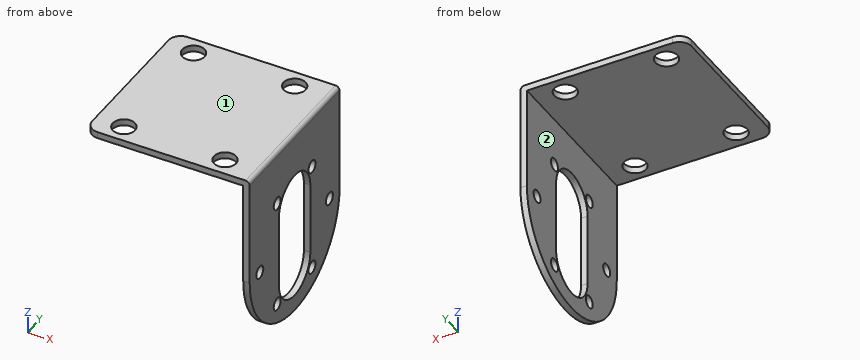
Autodesk Inventor part; units mm, degrees
ref_plane "작업 평면1" through (0, 0, 0) normal (0, 0, 1) x (1, 0, 0)
ref_plane "YZ Plane" through (0, 0, 0) normal (1, 0, 0) x (0, 1, 0)
ref_plane "XZ Plane" through (0, 0, 0) normal (0, 1, 0) x (-1, 0, 0)
ref_plane "작업 평면1" through (0, 0, 0) normal (0, 0, 1) x (1, 0, 0)
sketch "스케치1" plane through (0, 0, 0) normal (0, 0, 1) x (1, 0, 0)
  line L0 (130, -172.5) -> (91, -172.5)
  line L1 (91, -172.5) -> (91, -132.5)
  line L2 (91, -132.5) -> (130, -132.5)
  line L3 (130, -132.5) -> (130, -172.5)
  line L4 (91, -152.5) -> (130, -152.5) construction
  circle A0 centre (98, -168) radius 2.75
  line L5 (110.5, -172.5) -> (110.5, -132.5) construction
  circle A1 centre (98, -137) radius 2.75
  circle A2 centre (123, -168) radius 2.75
  circle A3 centre (123, -137) radius 2.75
  circle A4 centre (0, 170) radius 2
  circle A5 centre (-73.6122, 42.5) radius 2
  circle A6 centre (73.6122, 42.5) radius 2
  line L6 (-175, 220) -> (-175, 200)
  line L7 (-175, 200) -> (-130, 200)
  line L8 (-130, 200) -> (-130, 105)
  line L9 (-130, 105) -> (-175, 105)
  line L10 (-175, 105) -> (-175, -105)
  line L11 (-175, -105) -> (-130, -105)
  line L12 (-130, -105) -> (-130, -200)
  line L13 (-130, -200) -> (-175, -200)
  line L14 (-175, -200) -> (-175, -220)
  arc A7 (-175, -220) -> (-145, -250) centre (-145, -220) ccw
  line L15 (-145, -250) -> (145, -250)
  arc A8 (145, -250) -> (175, -220) centre (145, -220) ccw
  line L16 (175, -220) -> (175, -200)
  line L17 (175, -200) -> (130, -200)
  line L18 (130, -200) -> (130, -105)
  line L19 (130, -105) -> (175, -105)
  line L20 (175, -105) -> (175, 105)
  line L21 (175, 105) -> (130, 105)
  line L22 (130, 105) -> (130, 200)
  line L23 (130, 200) -> (175, 200)
  line L24 (175, 200) -> (175, 220)
  arc A9 (175, 220) -> (145, 250) centre (145, 220) ccw
  line L25 (145, 250) -> (-145, 250)
  arc A10 (-145, 250) -> (-175, 220) centre (-145, 220) ccw
  circle A11 centre (-123, 166.7672) radius 2
  circle A12 centre (122.9975, 135.7594) radius 2
  circle A13 centre (97.9975, -135.761) radius 2
  circle A14 centre (15.5, 71.3) radius 2
  circle A15 centre (165.0067, -210) radius 2.5
  circle A16 centre (119.0003, -180.2596) radius 1.25
  circle A17 centre (-119, -122.2672) radius 1.25
  circle A18 centre (-123, -135.7672) radius 2
  circle A19 centre (0.0196, 140) radius 2
  circle A20 centre (-123, -166.7672) radius 2
  circle A21 centre (-70, -122.2672) radius 1.25
  circle A22 centre (69.9966, -122.2627) radius 1.25
  circle A23 centre (-165, 0) radius 2.5
  circle A24 centre (-165.0067, 210) radius 2.5
  circle A25 centre (-15.5, 119.1) radius 2
  circle A26 centre (97.9995, -166.761) radius 2
  circle A27 centre (97.9995, 166.761) radius 2
  circle A28 centre (-98, 166.7672) radius 2
  circle A29 centre (-123, 135.7672) radius 2
  circle A30 centre (97.9975, 135.761) radius 2
  circle A31 centre (122.9975, -135.7594) radius 2
  circle A32 centre (-15.5, 71.3) radius 2
  circle A33 centre (-164.9933, -210) radius 2.5
  circle A34 centre (70.0003, -180.2627) radius 1.25
  circle A35 centre (-119, -180.2672) radius 1.25
  circle A36 centre (-98, -135.7672) radius 2
  circle A37 centre (47.6216, 57.483) radius 2
  circle A38 centre (-47.6412, 57.517) radius 2
  circle A39 centre (-98, -166.7672) radius 2
  circle A40 centre (-70, -180.2672) radius 1.25
  circle A41 centre (118.9966, -122.2596) radius 1.25
  circle A42 centre (165, 0) radius 2.5
  circle A43 centre (164.9933, 210) radius 2.5
  circle A44 centre (15.5, 119.1) radius 2
  circle A45 centre (122.9995, -166.7594) radius 2
  circle A46 centre (122.9995, 166.7594) radius 2
  circle A47 centre (-98, 135.7672) radius 2
  line L26 (-110, 97.5) -> (-93, 97.5)
  line L27 (-93, 97.5) -> (-93, 89.5)
  line L28 (-93, 89.5) -> (-110, 89.5)
  line L29 (-110, 89.5) -> (-110, 97.5)
  circle A48 centre (148, -23.75) radius 2
  circle A49 centre (130.626, -27.584) radius 1.5
  circle A50 centre (118.5, 61.5) radius 1.5
  circle A51 centre (-118.5, 61.5) radius 1.5
  circle A52 centre (21, -158.9548) radius 2
  circle A53 centre (-22, -53) radius 2
  circle A54 centre (-49.5, -194.9548) radius 2
  circle A55 centre (-49.5, -158.9548) radius 2
  circle A56 centre (21, -194.9548) radius 2
  circle A57 centre (-155, 25) radius 1.5
  circle A58 centre (118.5, 25) radius 1.5
  circle A59 centre (123.133, -76) radius 1.5
  circle A60 centre (37, -84) radius 2
  line L30 (-93, -89.5) -> (-93, -97.5)
  line L31 (-93, -97.5) -> (-110, -97.5)
  line L32 (-110, -97.5) -> (-110, -89.5)
  line L33 (-110, -89.5) -> (-93, -89.5)
  circle A61 centre (-130, 5) radius 6
  line L34 (110, 89.5) -> (93, 89.5)
  line L35 (93, 89.5) -> (93, 97.5)
  line L36 (93, 97.5) -> (110, 97.5)
  line L37 (110, 97.5) -> (110, 89.5)
  circle A62 centre (148, -84) radius 2
  circle A63 centre (47.999, -27.584) radius 1.5
  circle A64 centre (155, 61.5) radius 1.5
  circle A65 centre (-155, 61.5) radius 1.5
  circle A66 centre (49.5, -158.9548) radius 2
  circle A67 centre (-86, -93.5) radius 2
  circle A68 centre (-21, -194.9548) radius 2
  circle A69 centre (-150, -53) radius 2
  circle A70 centre (-21, -158.9548) radius 2
  circle A71 centre (49.5, -194.9548) radius 2
  circle A72 centre (-118.5, 25) radius 1.5
  circle A73 centre (155, 25) radius 1.5
  circle A74 centre (48, -76) radius 1.5
  circle A75 centre (37, -23.75) radius 2
  line L38 (110, -89.5) -> (110, -97.5)
  line L39 (110, -97.5) -> (93, -97.5)
  line L40 (93, -97.5) -> (93, -89.5)
  line L41 (93, -89.5) -> (110, -89.5)
  circle A76 centre (-70, 5) radius 6
  circle A77 centre (0, -216.4634) radius 1.5
  circle A78 centre (28.4775, -136.4634) radius 1.5
  circle A79 centre (-28.4775, -136.4634) radius 1.5
  point P0 (0, 0)
  dimension "d0" = 40
  dimension "d1" = 39
  dimension "d5" = 5.5
  dimension "d6" = 7
  dimension "d7" = 4.5
  dimension "d22" = 97.5
extrude "돌출1" add sketch "스케치1" along normal blind 1.6 contours L0 L1 L2 L3 | A0 A26 | A1 A13 | A2 A45 | A3 A31 picked at (98.3703, -165.1311) picked at (98.3657, -134.1305) picked at (122.627, -165.1309) picked at (123.3661, -134.13)
sketch "스케치2" plane through (130, -172.5, 0) normal (1, 0, 0) x (0, 0, -1)
  line L0 (0, 40) -> (-1.6, 40)
  line L1 (-1.6, 0) -> (25.4, 0)
  line L2 (45.4, 20) -> (45.4, 20)
  line L3 (25.4, 40) -> (-1.6, 40)
  line L4 (-1.6, 40) -> (-1.6, 0)
  arc A0 (25.4, 0) -> (45.4, 20) centre (25.4, 20) ccw
  arc A1 (45.4, 20) -> (25.4, 40) centre (25.4, 20) ccw
  circle A2 centre (25.4, 35.5) radius 1.55
  circle A3 centre (11.9766, 27.75) radius 1.55
  circle A4 centre (11.9766, 12.25) radius 1.55
  circle A5 centre (25.4, 4.5) radius 1.55
  circle A6 centre (38.8234, 12.25) radius 1.55
  circle A7 centre (38.8234, 27.75) radius 1.55
  line L5 (34.4, 20) -> (16.4, 20) construction
  line L6 (34.4, 27) -> (16.4, 27)
  line L7 (16.4, 13) -> (34.4, 13)
  arc A8 (34.4, 13) -> (34.4, 27) centre (34.4, 20) ccw
  arc A9 (16.4, 27) -> (16.4, 13) centre (16.4, 20) ccw
  line L8 (0, 40) -> (-1.6, 40)
  point P0 (0, 172.5)
  point P1 (45.4, 40)
  point P2 (45.4, 20)
  point P3 (-1.6, 40)
  point P4 (0, 40)
  dimension "d3" = 1.6
  dimension "d8" = 47
  dimension "d9" = 20
  dimension "d10" = 3.1
  dimension "d11" = 15.5
  dimension "d14" = 360
  dimension "d16" = 9
  dimension "d17" = 14
extrude "돌출2" add sketch "스케치2" along normal blind 1.6
fillet "모깎기1" radius 3 2 edges at (91, -132.5, 0.8) (91, -172.5, 0.8)
fillet "모깎기2" radius 1 1 edges at (131.6, -152.5, 1.6)
properties part number "SAFRS-P-0038"
Geometry: final body of the model. Coordinates: model frame, mm. Face numbers are marked on the shaded views. A direction names the side the tool comes from. Give positions to 0.01 mm unless a question says otherwise; leave off trailing zeros. Order: outer loops, then holes, each group sorted by start corner. A loop starts at its lowest first (then second) coordinate and runs counter-clockwise, first axis right, second up. Notation, with made-up numbers: (47, 48.25) -> (56, 48.25) arc R21 cw to (56, 70.25) -> close; hole circle Ø9 at (-28, 20). An arc over 180 degrees is marked (long way). Write each question's results on one line, items separated by ' | '. Start each with the question number.
1) Section A-A (x = 123). Return loops of the section in (y, z), then the cut area to 3 significant figures.
2) Section D-D (y = -161). Return loops of the section in (x, z), then the cut area to 3 significant figures.
3) Set-up query: the marked faces 1 and 2. Return all of +Z, -Z, +X, -X, +Y, -Y with unobstructed straight access to the full face (end or side cutting, diameter ignored); none if empty.
4) First-contact query: pin 1 (1.3 mm diameter, centred on x = 131, z = -27, fed in from +Y); pin 2 (1 mm diameter, centred on x = 124, y = -153, fed in from -Z); pin 3 (3.5 mm diameter, centred on y = -144.75, z = -11.98, fed in from -X). Flat tips, straight axial feed; report the tip coordinate or a pass-through.
5) Line query: line 1 (Y direction, x = 123, z = 1.05); line 2 (Z direction, x = 131, y = -144); line 3 (X direction, y = -134.5, z = -30). Output: solid intervals per line, ascending. Write a range as from..to.
6) Section B-B (z = -18). Return loops of the section in (x, y).
7) Section C-C (y = -152.5). Return loops of the section in (x, z), then the cut area to 3 significant figures.
Calculated:
1) outline: (-172.5, 0) -> (-170.75, 0) -> (-170.75, 1.6) -> (-172.5, 1.6) -> close; (-165.25, 0) -> (-139.75, 0) -> (-139.75, 1.6) -> (-165.25, 1.6) -> close; (-134.25, 0) -> (-132.5, 0) -> (-132.5, 1.6) -> (-134.25, 1.6) -> close | area: 46.4 mm2
2) outline: (91, 0) -> (130, 0) -> (130, -10.62) -> (131.6, -10.62) -> (131.6, 0.6) arc R1 ccw to (130.6, 1.6) -> (91, 1.6) -> close; (130, -43.5) -> (131.6, -43.5) -> (131.6, -40.18) -> (130, -40.18) -> close; (130, -37.47) -> (131.6, -37.47) -> (131.6, -13.33) -> (130, -13.33) -> close | area: 126 mm2
3) face 1: +Z, +X, -X, +Y, -Y | face 2: -Z, -X, +Y, -Y
4) pin 1: y = -132.52 | pin 2: z = 0 | pin 3: x = 130
5) line 1: -172.5..-170.75, -165.25..-139.75, -134.25..-132.5 | line 2: -43.5..-40.18, -37.47..-13.33, -10.62..1.52 | line 3: 130..131.6
6) outline: (130, -172.5) -> (131.6, -172.5) -> (131.6, -159.5) -> (130, -159.5) -> close; (130, -145.5) -> (131.6, -145.5) -> (131.6, -132.5) -> (130, -132.5) -> close
7) outline: (91, 0) -> (130, 0) -> (130, -9.4) -> (131.6, -9.4) -> (131.6, 0.6) arc R1 ccw to (130.6, 1.6) -> (91, 1.6) -> close; (130, -45.4) -> (131.6, -45.4) -> (131.6, -41.4) -> (130, -41.4) -> close | area: 86.2 mm2
